Could you check a few things on this model? Use its own coordinates, in mm. A direction names the side the tool comes from. Coordinates: 2 decimals unless noted, no trailing zeros. Loops run counter-clockwise (first coordinate to the right, second up) from the corner with the lowest first, then second, coordinate; pieces in that order, holes last.
from build123d import *

# Parameters (mm, degrees)
SKETCH_1_R          = 8.5
EXTRUDE_1_DEPTH     = 1.3
SKETCH_2_R          = 7.5
EXTRUDE_2_DEPTH     = 3.7
CUT_EXTRUDE_1_REACH = 15.019
SKETCH_3_R          = 3
SKETCH_4_R          = 6.25
SKETCH_4_R_2        = 4.25
CUT_EXTRUDE_2_DEPTH = 0.2
CUT_EXTRUDE_START   = -0.2
SKETCH_5_R          = 6.25
SKETCH_5_R_2        = 4.25
CUT_EXTRUDE_3_DEPTH = 0.2


with BuildPart() as part:
    # 草图1 → 凸台-拉伸1 (new body)
    with BuildSketch(Plane(origin=(0, 0, 0), x_dir=(1, 0, 0), z_dir=(0, 1, 0))):
        with Locations(Location((0, 0, 0), (0, 0, 270))):
            Circle(SKETCH_1_R)
    extrude(amount=EXTRUDE_1_DEPTH)

    # 草图2 → 凸台-拉伸2 (add)
    with BuildSketch(Plane(origin=(0, 1.3, 0), x_dir=(1, 0, 0), z_dir=(0, 1, 0))):
        with Locations(Location((0, 0, 0), (0, 0, 270))):
            Circle(SKETCH_2_R)
    extrude(amount=EXTRUDE_2_DEPTH)

    # 草图3 → 切除-拉伸1 (cut, up to next)
    with BuildSketch(Plane(origin=(0, 5, 0), x_dir=(1, 0, 0), z_dir=(0, 1, 0)), mode=Mode.PRIVATE) as cut_extrude_1_sk1:
        with Locations(Location((0, 0, 0), (0, 0, 270))):
            Circle(SKETCH_3_R)
    cut_extrude_1_tool1 = extrude(cut_extrude_1_sk1.sketch, amount=-CUT_EXTRUDE_1_REACH, mode=Mode.PRIVATE) & part.part
    add(cut_extrude_1_tool1.solids().sort_by_distance((0, 5, 0))[0], mode=Mode.SUBTRACT)

    # 草图4 → 切除-拉伸2 (cut)
    with BuildSketch(Plane(origin=(0, 5, 0), x_dir=(1, 0, 0), z_dir=(0, 1, 0))):
        with Locations(Location((0, 0, 0), (0, 0, 270))):
            Circle(SKETCH_4_R)
        with Locations(Location((0, 0, 0), (0, 0, 270))):
            Circle(SKETCH_4_R_2, mode=Mode.SUBTRACT)
    extrude(amount=-CUT_EXTRUDE_2_DEPTH, mode=Mode.SUBTRACT)

    # 草图5 → 切除-拉伸3 (cut)
    with BuildSketch(Plane.XZ.offset(CUT_EXTRUDE_START)):
        with Locations(Location((0, 0, 0), (0, 0, 90))):
            Circle(SKETCH_5_R)
        with Locations(Location((0, 0, 0), (0, 0, 90))):
            Circle(SKETCH_5_R_2, mode=Mode.SUBTRACT)
    extrude(amount=CUT_EXTRUDE_3_DEPTH, mode=Mode.SUBTRACT)


solid = part.part
(1) Imagine slicing it at C-C, the plane z = 7. Write out the boundary of the cut face in (x, y), and give its area (3 significant figures).
Answers:
outline: (-4.82, 0) - (4.82, 0) - (4.82, 1.3) - (2.69, 1.3) - (2.69, 5) - (-2.69, 5) - (-2.69, 1.3) - (-4.82, 1.3) - close
area: 32.5 mm2
(2) Imagine slicing it at B-B, the plane x = 0. Write out the boundary of the cut face in (y, z), and give its area (3 significant figures).
Answers:
outline: (0, -8.5) - (1.3, -8.5) - (1.3, -7.5) - (5, -7.5) - (5, -6.25) - (4.8, -6.25) - (4.8, -4.25) - (5, -4.25) - (5, -3) - (0, -3) - (0, -4.25) - (0.2, -4.25) - (0.2, -6.25) - (0, -6.25) - close; (0, 3) - (5, 3) - (5, 4.25) - (4.8, 4.25) - (4.8, 6.25) - (5, 6.25) - (5, 7.5) - (1.3, 7.5) - (1.3, 8.5) - (0, 8.5) - (0, 6.25) - (0.2, 6.25) - (0.2, 4.25) - (0, 4.25) - close
area: 46.0 mm2
(3) Imagine slicing it at A-A, the plane z = 0. Write out the boundary of the cut face in (x, y).
Answers:
outline: (-8.5, 0) - (-6.25, 0) - (-6.25, 0.2) - (-4.25, 0.2) - (-4.25, 0) - (-3, 0) - (-3, 5) - (-4.25, 5) - (-4.25, 4.8) - (-6.25, 4.8) - (-6.25, 5) - (-7.5, 5) - (-7.5, 1.3) - (-8.5, 1.3) - close; (3, 0) - (4.25, 0) - (4.25, 0.2) - (6.25, 0.2) - (6.25, 0) - (8.5, 0) - (8.5, 1.3) - (7.5, 1.3) - (7.5, 5) - (6.25, 5) - (6.25, 4.8) - (4.25, 4.8) - (4.25, 5) - (3, 5) - close
(4) Which directions (+Z, -Z, +X, -X, +Y, -Y) give clear straight access to the entire face, cutting with the end or side of a thin tool? Please do faces 1 (the face through (-1, 5, -3)), 2 (the face through (-8, 1.3, 0)).
Answers:
face 1: +Z, -Z, +X, -X, +Y
face 2: +Y
(5) Imagine slicing it at D-D, the plane z = 4.75. Write out the boundary of the cut face in (x, y).
Answers:
outline: (-7.05, 0) - (-4.06, 0) - (-4.06, 0.2) - (4.06, 0.2) - (4.06, 0) - (7.05, 0) - (7.05, 1.3) - (5.8, 1.3) - (5.8, 5) - (4.06, 5) - (4.06, 4.8) - (-4.06, 4.8) - (-4.06, 5) - (-5.8, 5) - (-5.8, 1.3) - (-7.05, 1.3) - close
(6) We'd pull the mould along Z, two halves only. Please class faces 3 (the face through (6, 5, -3)), 4 (the face through (0.9, 2.54, 2.86)), 5 (the face through (0.33, 3.124, -7.493)): +Z half, -Z half, draft (parallel to the pull), parting line (faces both ways), or undercut.
Answers:
face 3: draft
face 4: undercut
face 5: parting line
(7) For pin 1 (1.5 mm diameter, centred on x = 5, y = 3.5, fed in from +Z); pin 2 (1.5 mm diameter, centred on y = 3.5, z = -3.5, fed in from +X); pin 3 (3 mm diameter, centred on x = -0.5, y = 4, fed in from +Z), each with a flat end and sliding along its axis, tell me the tip position at first contact or that it passes through.
Answers:
pin 1: stops at z = 6.18
pin 2: stops at x = 6.98
pin 3: stops at z = 7.5
(8) I need wall thicknesses on probe 1 along X at (y, z) = (4.95, 0); probe 2 along X at (y, z) = (0.1, 0); probe 3 along Y at (x, z) = (7.25, -2.75). Which ranges of each line are inside material? Lowest first, please.
Answers:
probe 1: x = -7.5 to -6.25, -4.25 to -3, 3 to 4.25, 6.25 to 7.5
probe 2: x = -8.5 to -6.25, -4.25 to -3, 3 to 4.25, 6.25 to 8.5
probe 3: y = 0 to 1.3
